The listing builds one solid part. Answer for the finished solid, in the listing's coordinates (mm). Round coordinates to 2 decimals unless told otherwise and drop trailing zeros. Write each loop counter-clockwise with the first axis right and the second up, starting at its lowest first coordinate (ties: lowest second). Pieces come first, ordered by that corner, then holes.
(1) Find the intervals of material crossed by probe 1 along X at (y, z) = (34, 2.75); probe 2 along Z at (x, y) = (30, 64.5), in increasing order.
(2) The mould has two halves that part along X. Classify faces 1 (the face through (23.3, 66, 5)), 2 (the face through (37, 36, 8.5)), 3 (the face through (60.6, 35, 4)): +X half, -X half, draft (parallel to the pull), parting line (faces both ways), or undercut.
(3) A cutting plane is placed at C-C, the plane z = 7.5. Give the number of separate pieces and of enclosed holes in the cut face, and give its area (3 significant figures).
(4) A cutting plane is placed at B-B, the plane y = 45. Give the vertices of the cut face in (x, z).
(5) This flat-tipped pin is pushed along its axis until it touches: pin 1 Ø2.5 at (x, y) = (8.5, 65.5) entering from +Z. Where does it stop, or does it pass through?
from build123d import *

# Parameters (mm, degrees)
F0_W     = 60.6
F0_H     = 71.8
F1_DEPTH = 8.5
F2_W     = 56.6
F2_H     = 64.7999969125
F3_DEPTH = 6
F4_W     = 10
F4_H     = 7.5428567018
F5_DEPTH = 6


with BuildPart() as f1:
    # F0 (on Top) → F1 (new body)
    with BuildSketch(Plane.XY):
        with Locations((30.3, 35.9)):
            Rectangle(F0_W, F0_H)
    extrude(amount=F1_DEPTH)

    # F2 (on face) → F3 (cut)
    with BuildSketch(Plane.XY.offset(8.5)):
        with Locations((30.3, 37.3999984562)):
            Rectangle(F2_W, F2_H)
    extrude(amount=-F3_DEPTH, mode=Mode.SUBTRACT)

    # F4 (on face) → F5 (join)
    with BuildSketch(Plane.XY.offset(2.5)):
        Polygon((25.3, 69.7999969125), (23.3, 69.7999969125), (23.3, 62.2571402107), (2, 62.2571402107), (2, 60.2571402107), (23.3, 60.2571402107), (23.3, 52.7142835089), (2, 52.7142835089), (2, 50.7142835089), (23.3, 50.7142835089), (23.3, 43.1714268071), (2, 43.1714268071), (2, 41.1714268071), (23.3, 41.1714268071), (23.3, 33.6285701053), (2, 33.6285701053), (2, 31.6285701053), (23.3, 31.6285701053), (23.3, 24.0857134036), (2, 24.0857134036), (2, 22.0857134036), (23.3, 22.0857134036), (23.3, 14.5428567018), (2, 14.5428567018), (2, 12.5428567018), (23.3, 12.5428567018), (23.3, 5), (25.3, 5), (25.3, 12.5428567018), (35.3, 12.5428567018), (35.3, 5), (37.3, 5), (37.3, 12.5428567018), (58.6, 12.5428567018), (58.6, 14.5428567018), (37.3, 14.5428567018), (37.3, 22.0857134036), (58.6, 22.0857134036), (58.6, 24.0857134036), (37.3, 24.0857134036), (37.3, 31.6285701053), (58.6, 31.6285701053), (58.6, 33.6285701053), (37.3, 33.6285701053), (37.3, 41.1714268071), (58.6, 41.1714268071), (58.6, 43.1714268071), (37.3, 43.1714268071), (37.3, 50.7142835089), (58.6, 50.7142835089), (58.6, 52.7142835089), (37.3, 52.7142835089), (37.3, 60.2571402107), (58.6, 60.2571402107), (58.6, 62.2571402107), (37.3, 62.2571402107), (37.3, 69.7999969125), (35.3, 69.7999969125), (35.3, 62.2571402107), (25.3, 62.2571402107), align=None)
        with Locations((30.3, 18.3142850527)):
            Rectangle(F4_W, F4_H, mode=Mode.SUBTRACT)
        with Locations((30.3, 27.8571417545)):
            Rectangle(F4_W, F4_H, mode=Mode.SUBTRACT)
        with Locations((30.3, 37.3999984562)):
            Rectangle(F4_W, F4_H, mode=Mode.SUBTRACT)
        with Locations((30.3, 46.942855158)):
            Rectangle(F4_W, F4_H, mode=Mode.SUBTRACT)
        with Locations((30.3, 56.4857118598)):
            Rectangle(F4_W, F4_H, mode=Mode.SUBTRACT)
    extrude(amount=F5_DEPTH)


with BuildPart() as f6_1:
    # F6: copy of F1
    add(f1.part)


solid = f1.part
Solutions:
1. probe 1: x = 0 to 2, 23.3 to 25.3, 35.3 to 37.3, 58.6 to 60.6
1. probe 2: z = 0 to 2.5
2. face 1: undercut
2. face 2: draft
2. face 3: +X half
3. separate pieces: 1
3. enclosed holes: 21
3. area: 1,570 mm2
4. outline: (0, 0) - (60.6, 0) - (60.6, 8.5) - (58.6, 8.5) - (58.6, 2.5) - (37.3, 2.5) - (37.3, 8.5) - (35.3, 8.5) - (35.3, 2.5) - (25.3, 2.5) - (25.3, 8.5) - (23.3, 8.5) - (23.3, 2.5) - (2, 2.5) - (2, 8.5) - (0, 8.5) - close
5. pin 1: stops at z = 2.5
